Design review of the part shown in the three views and the two pictorial views. Dimensions are in mm from the part's minimum x, y and z. Give positions to 0.01 mm unless a question says otherwise; leave off trailing zeros. Loops run counter-clockwise (first coordinate to the right, second up) from the corner with the lowest first, then second, coordinate; pieces in that order, holes last. Notation, with made-up numbers: (36, 66) -> (65, 66) arc R17 ccw to (65, 83) -> close; hole circle Ø4 at (53.5, 59). An arc over 180 degrees is marked (long way). Use CSV: the item, a comma, the result in double quotes. Start each with the question number.
Item 1: Wall thickness on line 1 along X through (y, z) = (24.5, 17); line 2 along Z through (x, y) = (56, 15.5); line 3 along Y through (x, z) = (431.5, 20): over which ranges is each line inside the solid? List them lowest first. Write a range as from..to.
Item 2: Clearance check with flat-ended pins moving along their axes: pin 1 (10 mm diameter, centred on x = 211, y = 11.5, fed in from +Z); pin 2 (7.5 mm diameter, centred on x = 64, z = 20, fed in from +Y); pin 3 (10 mm diameter, centred on x = 94.5, y = 24.5, fed in from +Z). State where each tip first meets the part, or that it passes through.
Item 3: We need section C-C (x = 52.5). State the section outline as (y, z) points, plus the area to 3 significant figures.
Item 4: We need section B-B (y = 15). State the section outline as (x, z) points.
Item 5: We need section A-A (z = 25.5). State the section outline as (x, y) points.
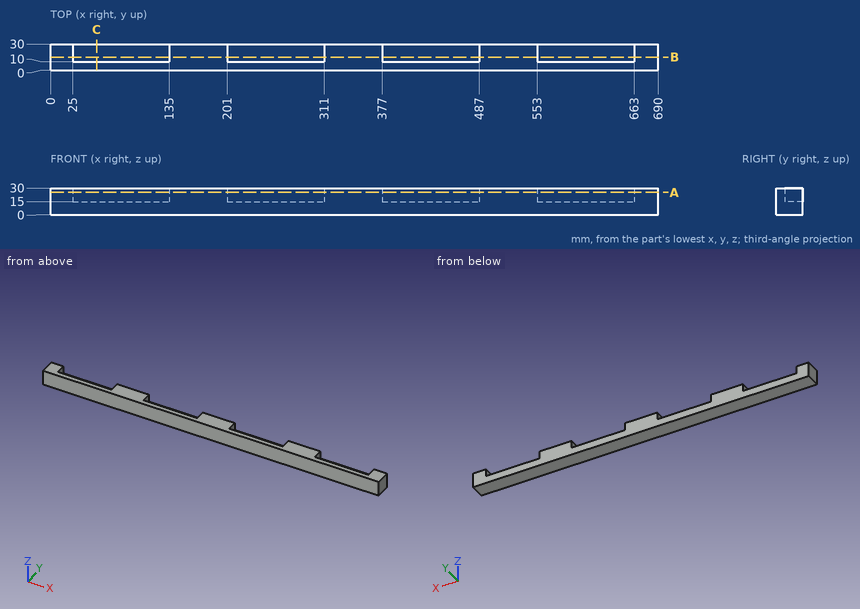
Results found:
1,line 1,"0..25, 135..201, 311..377, 487..553, 663..690"
1,line 2,"0..15"
1,line 3,"0..10"
2,pin 1,"z = 30"
2,pin 2,"y = 10"
2,pin 3,"z = 15"
3,outline,"(0, 0) -> (30, 0) -> (30, 15) -> (10, 15) -> (10, 30) -> (0, 30) -> close"
3,area,"600 mm²"
4,outline,"(0, 0) -> (690, 0) -> (690, 30) -> (663, 30) -> (663, 15) -> (553, 15) -> (553, 30) -> (487, 30) -> (487, 15) -> (377, 15) -> (377, 30) -> (311, 30) -> (311, 15) -> (201, 15) -> (201, 30) -> (135, 30) -> (135, 15) -> (25, 15) -> (25, 30) -> (0, 30) -> close"
5,outline,"(0, 0) -> (690, 0) -> (690, 30) -> (663, 30) -> (663, 10) -> (553, 10) -> (553, 30) -> (487, 30) -> (487, 10) -> (377, 10) -> (377, 30) -> (311, 30) -> (311, 10) -> (201, 10) -> (201, 30) -> (135, 30) -> (135, 10) -> (25, 10) -> (25, 30) -> (0, 30) -> close"
